```python
from build123d import *

# Parameters (mm, degrees)
SKETCH_1_R      = 11.5
SKETCH_1_R_2    = 1.5
EXTRUDE_1_DEPTH = 5


with BuildPart() as part:
    # 草图1 → 凸台-拉伸1 (new body)
    with BuildSketch(Plane.XY):
        Polygon((0, 40), (0, 60), (60, 60), (60, 40), (55, 40), (55, 20), (60, 20), (60, 0), (45, 0), (45, -5), (15, -5), (15, 0), (0, 0), (0, 20), (5, 20), (5, 40), align=None)
        with Locations((30, 30)):
            Circle(SKETCH_1_R, mode=Mode.SUBTRACT)
        with Locations((14.5, 45.5)):
            Circle(SKETCH_1_R_2, mode=Mode.SUBTRACT)
        with Locations((45.5, 45.5)):
            Circle(SKETCH_1_R_2, mode=Mode.SUBTRACT)
        with Locations((45.5, 14.5)):
            Circle(SKETCH_1_R_2, mode=Mode.SUBTRACT)
        with Locations((14.5, 14.5)):
            Circle(SKETCH_1_R_2, mode=Mode.SUBTRACT)
    extrude(amount=EXTRUDE_1_DEPTH)


solid = part.part
```
Geometry check sheet. Reference: the model listing, model coordinates, mm. A direction names the side the tool comes from. Round coordinates to 2 decimals unless told otherwise and drop trailing zeros. Order: outer loops, then holes, each group sorted by start corner. A loop starts at its lowest first (then second) coordinate and runs counter-clockwise, first axis right, second up. Notation, with made-up numbers: (38.25, -17) -> (89.25, -17) arc R33 ccw to (89.25, 17) -> close; hole circle Ø7 at (86.5, 1.5). An arc over 180 degrees is marked (long way). Return JSON: item names as keys, results as strings. Group by question number.
Q1. Section check C-C, the plane y = 14.5. Record the boundary of the cut face in (x, z), plus the area to 3 significant figures.
Q2. Release check for a two-part mould opening along X. For faces 6 (the flat face through (5, 30, 2)), 7 (the flat face through (30, -5, 2)), 8 (the cylindrical face through (20.874, 23.002, 2.465)) record: released by +X, released by -X, zero draft, split by the parting line, or undercut.
Q3. Material ranges on probe 1 along Y at (x, z) = (45.5, 3.5); probe 2 along X at (y, z) = (13.5, 3.2); probe 3 along Y at (x, z) = (14, 4.65), recorded low to high. Write a range as from..to.
Q4. Section check B-B, the plane z = 4.25. Record the boundary of the cut face in (x, y).
Q5. Gauge pin test, flat ends, axial feed: pin 1 (2.5 mm diameter, centred on y = -3, z = 1.5, fed in from -X); pin 2 (2.5 mm diameter, centred on x = 58.5, z = 3, fed in from -Y); pin 3 (2.5 mm diameter, centred on x = 14.5, y = 45.5, fed in from -Z); pin 4 (5 mm diameter, centred on x = 45.5, y = 45.5, fed in from +Z). Record the tip position at first contact, or that the pin passes through.
Q6. Tool access check on faces 1 (the flat face through (37.1, 20.7, 5)), 2 (the flat face through (55, 30, 2)), 3 (the flat face through (3, 40, 2)), 4 (the flat face through (53, 0, 2)), 5 (the flat face through (8, 0, 2)). Record the directions out of +Z, -Z, +X, -X, +Y, -Y that give a thin tool (end or side, any length) a straight path to the whole face; none if there is none.
Q7. Section check A-A, the plane x = 30. Record the boundary of the cut face in (y, z), plus the area to 3 significant figures.
Q8. Section check D-D, the plane y = 26.5. Record the boundary of the cut face in (x, z).
Numbers:
{
 "1": {"outline": "(0, 0) -> (13, 0) -> (13, 5) -> (0, 5) -> close; (16, 0) -> (44, 0) -> (44, 5) -> (16, 5) -> close; (47, 0) -> (60, 0) -> (60, 5) -> (47, 5) -> close", "area": "270 mm^2"},
 "2": {"face 6": "released by -X", "face 7": "zero draft", "face 8": "undercut"},
 "3": {"probe 1": "0..13, 16..44, 47..60", "probe 2": "0..13.38, 15.62..44.38, 46.62..60", "probe 3": "0..13.09, 15.91..44.09, 46.91..60"},
 "4": {"outline": "(0, 0) -> (15, 0) -> (15, -5) -> (45, -5) -> (45, 0) -> (60, 0) -> (60, 20) -> (55, 20) -> (55, 40) -> (60, 40) -> (60, 60) -> (0, 60) -> (0, 40) -> (5, 40) -> (5, 20) -> (0, 20) -> close; hole circle Ø3 at (14.5, 14.5); hole circle Ø3 at (14.5, 45.5); hole circle Ø23 at (30, 30); hole circle Ø3 at (45.5, 14.5); hole circle Ø3 at (45.5, 45.5)"},
 "5": {"pin 1": "x = 15", "pin 2": "y = 0", "pin 3": "through", "pin 4": "z = 5"},
 "6": {"face 1": "+Z, +X, -X, +Y, -Y", "face 2": "+Z, -Z, +X", "face 3": "+Z, -Z, -X", "face 4": "+Z, -Z, +X, -Y", "face 5": "+Z, -Z, -X, -Y"},
 "7": {"outline": "(-5, 0) -> (18.5, 0) -> (18.5, 5) -> (-5, 5) -> close; (41.5, 0) -> (60, 0) -> (60, 5) -> (41.5, 5) -> close", "area": "210 mm^2"},
 "8": {"outline": "(5, 0) -> (19.05, 0) -> (19.05, 5) -> (5, 5) -> close; (40.95, 0) -> (55, 0) -> (55, 5) -> (40.95, 5) -> close"}
}
